For this review, take the finished solid that the model builds, in its own axes (mm). Face numbers are marked on the shaded views. A direction names the side the tool comes from. Give positions to 0.01 mm unless a question says otherwise; leave off trailing zeros. Order: outer loops, then holes, each group sorted by start corner. A loop starts at its lowest first (then second) coordinate and runs counter-clockwise, first axis right, second up.
Item 1: For P1, Ø6, axis at x = -14.5, z = 8.5, coming from the -Y side; P2, Ø1.5, axis at x = 34, z = 23, coming from the -Y side, all flat-tipped, find the tip position at first contact; note any pin that passes through.
Item 2: Consider section C-C (z = 23.5). Give the boundary of the cut face in (x, y).
Item 3: The part is to be moulded in two halves that separate along Z. For the marked faces 3, 4 and 5, say which applies: released by +Z, released by -Z, zero draft, split by the parting line, or undercut.
Item 4: Consider section B-B (x = -31.5). Give the boundary of the cut face in (y, z), plus the area to 3 significant figures.
Item 5: Machinability: for the marked faces 1 and 2, which of the approach directions +Z, -Z, +X, -X, +Y, -Y give a long, thin tool a straight path to every point of the face, cutting with its end or side? Answer none if there is none.
Item 6: For probe 1 along X at (y, z) = (-3.75, -6.5); probe 2 along Z at (x, y) = (22, -9.25); probe 3 along Z at (x, y) = (33.5, -4.5), list the stretches that pass through material, from the lowest coordinate up.
Item 7: Consider section A-A (y = -15.25). Give the boundary of the cut face in (x, z), plus the area to 3 significant figures.
Item 8: Consider section D-D (x = 34.5). Give the boundary of the cut face in (y, z), plus the area to 3 significant figures.
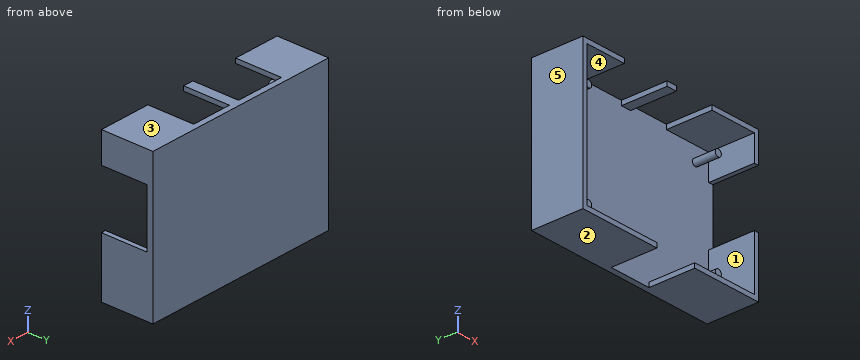
```python
from build123d import *

# Parameters (mm, degrees)
F0_W     = 86
F0_H     = 64
F0_W_2   = 82
F0_H_2   = 60
F0_R     = 1.5
F1_DEPTH = 2.5
F2_DEPTH = 10
F3_DEPTH = 20
F4_W     = 20
F4_H     = 25
F5_DEPTH = 2
F6_W     = 18.5
F6_H     = 20
F7_DEPTH = 2
F8_W     = 21
F8_H     = 20
F8_W_2   = 17.5
F9_DEPTH = 2


with BuildPart() as f1:
    # F0 (on Front) → F1 (new body)
    with BuildSketch(Plane.XZ):
        Rectangle(F0_W, F0_H)
        Rectangle(F0_W_2, F0_H_2, mode=Mode.SUBTRACT)
        Rectangle(F0_W_2, F0_H_2)
        with Locations((-29, -21)):
            Circle(F0_R, mode=Mode.SUBTRACT)
        with Locations((34.5, -21)):
            Circle(F0_R, mode=Mode.SUBTRACT)
        with Locations((-29, 23.5)):
            Circle(F0_R, mode=Mode.SUBTRACT)
        with Locations((34.5, 23.5)):
            Circle(F0_R, mode=Mode.SUBTRACT)
        with Locations((-29, 23.5)):
            Circle(F0_R)
        with Locations((-29, -21)):
            Circle(F0_R)
        with Locations((34.5, -21)):
            Circle(F0_R)
        with Locations((34.5, 23.5)):
            Circle(F0_R)
    extrude(amount=-F1_DEPTH)

    # F0 (on Front) → F2 (join)
    with BuildSketch(Plane.XZ):
        with Locations((-29, 23.5)):
            Circle(F0_R)
        with Locations((-29, -21)):
            Circle(F0_R)
        with Locations((34.5, -21)):
            Circle(F0_R)
        with Locations((34.5, 23.5)):
            Circle(F0_R)
    extrude(amount=F2_DEPTH)

    # F0 (on Front) → F3 (join)
    with BuildSketch(Plane.XZ):
        Rectangle(F0_W, F0_H)
        Rectangle(F0_W_2, F0_H_2, mode=Mode.SUBTRACT)
    extrude(amount=F3_DEPTH)

    # F4 (on face) → F5 (cut)
    with BuildSketch(Plane.YZ.offset(43)):
        with Locations((-10, 6.25)):
            Rectangle(F4_W, F4_H)
    extrude(amount=-F5_DEPTH, mode=Mode.SUBTRACT)

    # F6 (on face) → F7 (cut)
    with BuildSketch(Plane(origin=(0, 0, -32), x_dir=(1, 0, 0), z_dir=(0, 0, -1))):
        with Locations((2.5, 10)):
            Rectangle(F6_W, F6_H)
    extrude(amount=-F7_DEPTH, mode=Mode.SUBTRACT)

    # F8 (on face) → F9 (cut)
    with BuildSketch(Plane.XY.offset(32)):
        with Locations((-12.25, -10)):
            Rectangle(F8_W, F8_H)
        with Locations((11.5, -10)):
            Rectangle(F8_W_2, F8_H)
    extrude(amount=-F9_DEPTH, mode=Mode.SUBTRACT)


solid = f1.part
```
Resolved:
1. P1: stops at y = 0
1. P2: stops at y = -10
2. outline: (-43, -20) - (-41, -20) - (-41, 0) - (-30.5, 0) - (-30.5, -10) - (-27.5, -10) - (-27.5, 0) - (33, 0) - (33, -10) - (36, -10) - (36, 0) - (41, 0) - (41, -20) - (43, -20) - (43, 2.5) - (-43, 2.5) - close
3. face 3: released by +Z
3. face 4: undercut
3. face 5: zero draft
4. outline: (-20, -32) - (2.5, -32) - (2.5, 32) - (-20, 32) - (-20, 30) - (0, 30) - (0, -30) - (-20, -30) - close
4. area: 240 mm2
5. face 1: -Y
5. face 2: -Z, +X, -X, +Y, -Y
6. probe 1: x = -43 to -41, 41 to 43
6. probe 2: z = -32 to -30, 30 to 32
6. probe 3: z = -32 to -30, -22.12 to -19.88, 22.38 to 24.62, 30 to 32
7. outline: (-43, -32) - (-6.75, -32) - (-6.75, -30) - (-41, -30) - (-41, 30) - (-22.75, 30) - (-22.75, 32) - (-43, 32) - close; (-1.75, 30) - (2.75, 30) - (2.75, 32) - (-1.75, 32) - close; (11.75, -32) - (43, -32) - (43, -6.25) - (41, -6.25) - (41, -30) - (11.75, -30) - close; (20.25, 30) - (41, 30) - (41, 18.75) - (43, 18.75) - (43, 32) - (20.25, 32) - close
7. area: 420 mm2
8. outline: (-20, -32) - (2.5, -32) - (2.5, 32) - (-20, 32) - (-20, 30) - (0, 30) - (0, 25) - (-10, 25) - (-10, 22) - (0, 22) - (0, -19.5) - (-10, -19.5) - (-10, -22.5) - (0, -22.5) - (0, -30) - (-20, -30) - close
8. area: 300 mm2
